```python
from build123d import *

# Parameters (mm, degrees)
SKETCH_1_R               = 1.5
EXTRUDE_1_DEPTH          = 55
SKETCH_2_R               = 12
EXTRUDE_2_DEPTH          = 80
CUT_EXTRUDE_START        = -40
CUT_EXTRUDE_1_DEPTH      = 40
CUT_EXTRUDE_2_DEPTH      = 97.710909566
CUT_EXTRUDE_2_DEPTH_BACK = 97.710909566
SKETCH_5_R               = 2


with BuildPart() as part:
    # 草图1 → 凸台-拉伸1 (new body)
    with BuildSketch(Plane(origin=(0, 0, 0), x_dir=(1, 0, 0), z_dir=(0, 1, 0))):
        with Locations(Location((0, 0, 0), (0, 0, 270))):
            Circle(SKETCH_1_R)
    extrude(amount=EXTRUDE_1_DEPTH)

    # 草图2 → 凸台-拉伸2 (add)
    with BuildSketch(Plane(origin=(0, 0, 0), x_dir=(0, 0, -1), z_dir=(1, 0, 0))):
        with Locations(Location((0, 0, 0), (0, 0, 97.180755781))):
            Circle(SKETCH_2_R)
    extrude(amount=EXTRUDE_2_DEPTH)

    # 草图4 → 切除-拉伸1 (cut)
    with BuildSketch(Plane(origin=(80, 0, 0), x_dir=(0, 0, -1), z_dir=(1, 0, 0)).offset(CUT_EXTRUDE_START)):
        with BuildLine():
            Line((-11.832159566, -2), (-10.908712115, -2))
            Line((-10.908712115, -2), (10.908712115, -2))
            Line((10.908712115, -2), (11.832159566, -2))
            ThreePointArc((11.832159566, -2), (11.957966273, -1.003515123), (12, 0))
            ThreePointArc((12, 0), (11.957966273, 1.003515123), (11.832159566, 2))
            Line((11.832159566, 2), (-6.712374636, 2))
            Line((-6.712374636, 2), (-11.832159566, 2))
            ThreePointArc((-11.832159566, 2), (-12, 0), (-11.832159566, -2))
        make_face()
    extrude(amount=CUT_EXTRUDE_1_DEPTH, mode=Mode.SUBTRACT)

    # 草图5 → 切除-拉伸2 (cut, two sides: drawn at the far end of the back side and taken through both)
    with BuildSketch(Plane.XZ.offset(-2).offset(-CUT_EXTRUDE_2_DEPTH_BACK)):
        with Locations(Location((70, 0, 0), (0, 0, 270))):
            Circle(SKETCH_5_R)
    extrude(amount=CUT_EXTRUDE_2_DEPTH + CUT_EXTRUDE_2_DEPTH_BACK, mode=Mode.SUBTRACT)


solid = part.part
```
Design review of the part built by this model. Coordinates are the model's own, in mm. A direction names the side the tool comes from. Coordinates: 2 decimals unless noted, no trailing zeros. Loops run counter-clockwise (first coordinate to the right, second up) from the corner with the lowest first, then second, coordinate; pieces in that order, holes last. Notation, with made-up numbers: (42, 69) - (74, 69) arc R8 ccw to (74, 79) - close; hole circle Ø11 at (44.5, -21). An arc over 180 degrees is marked (long way). Use CSV: the item, a comma, the result in double quotes. Start each with the question number.
1) Wall thickness on L1, parallel to Y at x = 62.5, z = 2; L2, parallel to X at y = -6.25, z = 0; L3, parallel to Y at x = 74.5, z = 0.5: over which ranges is each line inside the solid? List them lowest first. Write a range as from..to.
2) For pin 1 Ø7 at (x, z) = (54.5, -5) entering from +Y; pin 2 Ø1 at (x, z) = (44, 7) entering from -Y; pin 3 Ø3 at (x, z) = (19.5, 9) entering from +Y, all flat-tipped, find the tip position at first contact; note any pin that passes through.
3) The part is to be moulded in two halves that separate along X. For faces 1 (the cylindrical face through (72, -7, 0)), 2 (the flat face through (40, 0, 0)), 3 (the cylindrical face through (-1.464, 27.115, -0.325)), say which applies: +X half, -X half, draft (parallel to the pull), parting line (faces both ways), or undercut.
4) Consider section D-D on y = 6. Write out the cut boundary in (x, z).
5) Consider section A-A on x = 70. Write out the cut boundary in (y, z).
6) Tool access review of faces 4 (the flat face through (60, 2, 0)), 5 (the flat face through (0, 55, 0)): name each direction out of +Z, -Z, +X, -X, +Y, -Y from which nothing blocks a thin tool from reaching the whole face with its end or side.
7) Consider section C-C on z = 10.25. Write out the cut boundary in (x, y), then the cut area to 3 significant figures.
8) Consider section B-B on z = 0. Write out the cut boundary in (x, y).
Geometry says:
1,L1,"-11.83..-2, 2..11.83"
1,L2,"0..68, 72..80"
1,L3,"-11.99..-2, 2..11.99"
2,pin 1,"y = 11.91"
2,pin 2,"y = -10.09"
2,pin 3,"y = 9.37"
3,face 1,"undercut"
3,face 2,"+X half"
3,face 3,"parting line"
4,outline,"(0, -10.39) - (80, -10.39) - (80, 10.39) - (0, 10.39) - (0, 1.5) arc R1.5 ccw to (0, -1.5) - close; hole circle Ø4 at (70, 0)"
5,outline,"(-11.83, -2) arc R12 ccw to (-2, -11.83) - (-2, -2) - close; (-11.83, 2) - (-2, 2) - (-2, 11.83) arc R12 ccw to start; (2, -11.83) arc R12 ccw to (11.83, -2) - (2, -2) - close; (2, 2) - (11.83, 2) arc R12 ccw to (2, 11.83) - close"
6,face 4,"+Z, -Z, +X"
6,face 5,"+Z, -Z, +X, -X, +Y"
7,outline,"(0, -6.24) - (80, -6.24) - (80, -2) - (40, -2) - (40, 2) - (80, 2) - (80, 6.24) - (0, 6.24) - close"
7,area,"838 mm^2"
8,outline,"(-1.5, 0) - (0, 0) - (0, -12) - (68, -12) - (68, -2) - (40, -2) - (40, 2) - (68, 2) - (68, 12) - (1.5, 12) - (1.5, 55) - (-1.5, 55) - close; (72, -12) - (80, -12) - (80, -2) - (72, -2) - close; (72, 2) - (80, 2) - (80, 12) - (72, 12) - close"
